from build123d import *

# Parameters (mm, degrees)
SKETCH1_W           = 20
SKETCH1_H           = 25
SKETCH1_W_2         = 25
SKETCH1_H_2         = 20
BOSS_EXTRUDE1_DEPTH = 10
SKETCH2_R           = 2.5
CUT_EXTRUDE1_DEPTH  = 57.402570863
SKETCH3_R           = 2.5
CUT_EXTRUDE2_DEPTH  = 57.402570863
SKETCH4_R           = 2.5
BOSS_EXTRUDE2_DEPTH = 40
SKETCH5_W           = 1
SKETCH5_H           = 3


with BuildPart() as part:
    # Sketch1 → Boss-Extrude1 (new body)
    with BuildSketch(Plane(origin=(0, 0, 0), x_dir=(1, 0, 0), z_dir=(0, 1, 0))):
        with Locations((-22.5, 0)):
            Rectangle(SKETCH1_W, SKETCH1_H)
        with Locations((0, -22.5)):
            Rectangle(SKETCH1_W_2, SKETCH1_H_2)
        Rectangle(SKETCH1_W_2, SKETCH1_H)
        with Locations((0, 22.5)):
            Rectangle(SKETCH1_W_2, SKETCH1_H_2)
        with Locations((22.5, 0)):
            Rectangle(SKETCH1_W, SKETCH1_H)
    extrude(amount=BOSS_EXTRUDE1_DEPTH)

    # Sketch2 → Cut-Extrude1 (cut, through all)
    with BuildSketch(Plane(origin=(12.5, 0, 0), x_dir=(0, 0, -1), z_dir=(1, 0, 0))):
        with Locations((-26.499999999, 5)):
            Circle(SKETCH2_R)
        with Locations((26.499999999, 5)):
            Circle(SKETCH2_R)
    extrude(amount=-CUT_EXTRUDE1_DEPTH, mode=Mode.SUBTRACT)

    # Sketch3 → Cut-Extrude2 (cut, through all)
    with BuildSketch(Plane.XY.offset(12.5)):
        with Locations((26.5, 5)):
            Circle(SKETCH3_R)
        with Locations((-26.5, 5)):
            Circle(SKETCH3_R)
    extrude(amount=-CUT_EXTRUDE2_DEPTH, mode=Mode.SUBTRACT)

    # Sketch4 → Boss-Extrude2 (add)
    with BuildSketch(Plane(origin=(0, 0, 0), x_dir=(1, 0, 0), z_dir=(0, 1, 0))):
        with Locations(Location((0, 0, 0), (0, 0, 270))):
            Circle(SKETCH4_R)
    extrude(amount=-BOSS_EXTRUDE2_DEPTH)

    # Sketch5 → Cut-Revolve1 (revolve, cut)
    with BuildSketch(Plane(origin=(0, 0, 0), x_dir=(0, 0, -1), z_dir=(1, 0, 0)), mode=Mode.PRIVATE) as cut_revolve1_sk:
        with Locations((2, -30.5)):
            Rectangle(SKETCH5_W, SKETCH5_H)
    revolve(cut_revolve1_sk.sketch.rotate(Axis((0, 0, 0), (0, -1, 0)), 180), axis=Axis((0, 0, 0), (0, -1, 0)), mode=Mode.SUBTRACT)


solid = part.part
Work out the finished part from the listing and answer in its coordinate system (mm). A direction names the side the tool comes from. Give positions to 0.01 mm unless a question says otherwise; leave off trailing zeros. Write each loop counter-clockwise with the first axis right and the second up, starting at its lowest first coordinate (ties: lowest second). Pieces come first, ordered by that corner, then holes. Notation, with made-up numbers: (5.5, 56.5) - (28.5, 56.5) arc R17 cw to (28.5, 72.5) - close; hole circle Ø4 at (6.25, -5). An arc over 180 degrees is marked (long way). One line per item, written item: value. Start each with the question number.
1. For faces 1 (the flat face through (-12.5, 5, 23)), 2 (the flat face through (12.5, 5, 23)), 3 (the cylindrical face through (-2.44, -14.3, -0.54)), determine the directions among +Z, -Z, +X, -X, +Y, -Y from which every point of the face is accessible in a straight line to the end or side of a thin tool.
2. Given pin 1 (8 mm diameter, centred on y = 6.5, z = 18, fed in from -X); pin 2 (3 mm diameter, centred on x = -5.5, z = 0, fed in from -Y); pin 3 (4.5 mm diameter, centred on x = -26.5, y = 5, fed in from +Z); pin 4 (11 mm diameter, centred on y = 4.5, z = -20.5, fed in from +X), each flat-ended and moving along its own axis, determine where each tip first touches the part or whether it passes through.
3. Find section A-A (z = 26.5). Write down the section's boundary in (x, y), then the cut area to 3 significant figures.
4. Find section C-C (x = 26.5). Write down the section's boundary in (y, z), then the cut area to 3 significant figures.
5. Consider probe 1 along Y at (x, z) = (26.5, 1.5); probe 2 along Z at (x, y) = (4.5, 4.5); probe 3 along Y at (x, z) = (-23, 8.5). Determine where each line is inside the solid, lowest interval first.
6. Find section D-D (x = 6). Write down the section's boundary in (y, z).
7. Find section B-B (y = 5). Write down the section's boundary in (x, z), then the cut area to 4 significant figures.
8. For a pull along Z with two mould halves and no side action, classify faces 4 (the flat face through (-22, 5, -12.5)), 5 (the cylindrical face through (0.175, 5.751, 24.115)), 6 (the flat face through (-12.5, 5, -22)) as +Z half, -Z half, draft (parallel to the pull), parting line (faces both ways), or undercut.
Geometry results:
1. face 1: +Z, -X, +Y, -Y
1. face 2: +Z, +X, +Y, -Y
1. face 3: -Y
2. pin 1: x = -12.5
2. pin 2: y = 0
2. pin 3: through
2. pin 4: x = 12.5
3. outline: (-12.5, 0) - (12.5, 0) - (12.5, 2.5) - (-12.5, 2.5) - close; (-12.5, 7.5) - (12.5, 7.5) - (12.5, 10) - (-12.5, 10) - close
3. area: 125 mm2
4. outline: (0, -12.5) - (2.5, -12.5) - (2.5, 12.5) - (0, 12.5) - close; (7.5, -12.5) - (10, -12.5) - (10, 12.5) - (7.5, 12.5) - close
4. area: 125 mm2
5. probe 1: 0 to 2.5, 7.5 to 10
5. probe 2: -32.5 to -28.95, -24.05 to 24.05, 28.95 to 32.5
5. probe 3: 0 to 10
6. outline: (0, -32.5) - (10, -32.5) - (10, 32.5) - (0, 32.5) - close; hole circle Ø5 at (5, -26.5); hole circle Ø5 at (5, 26.5)
7. outline: (-32.5, -12.5) - (-29, -12.5) - (-29, 12.5) - (-32.5, 12.5) - close; (-24, -12.5) - (-12.5, -12.5) - (-12.5, -24) - (12.5, -24) - (12.5, -12.5) - (24, -12.5) - (24, 12.5) - (12.5, 12.5) - (12.5, 24) - (-12.5, 24) - (-12.5, 12.5) - (-24, 12.5) - close; (-12.5, -32.5) - (12.5, -32.5) - (12.5, -29) - (-12.5, -29) - close; (-12.5, 29) - (12.5, 29) - (12.5, 32.5) - (-12.5, 32.5) - close; (29, -12.5) - (32.5, -12.5) - (32.5, 12.5) - (29, 12.5) - close
7. area: 2,125 mm2
8. face 4: -Z half
8. face 5: undercut
8. face 6: draft
